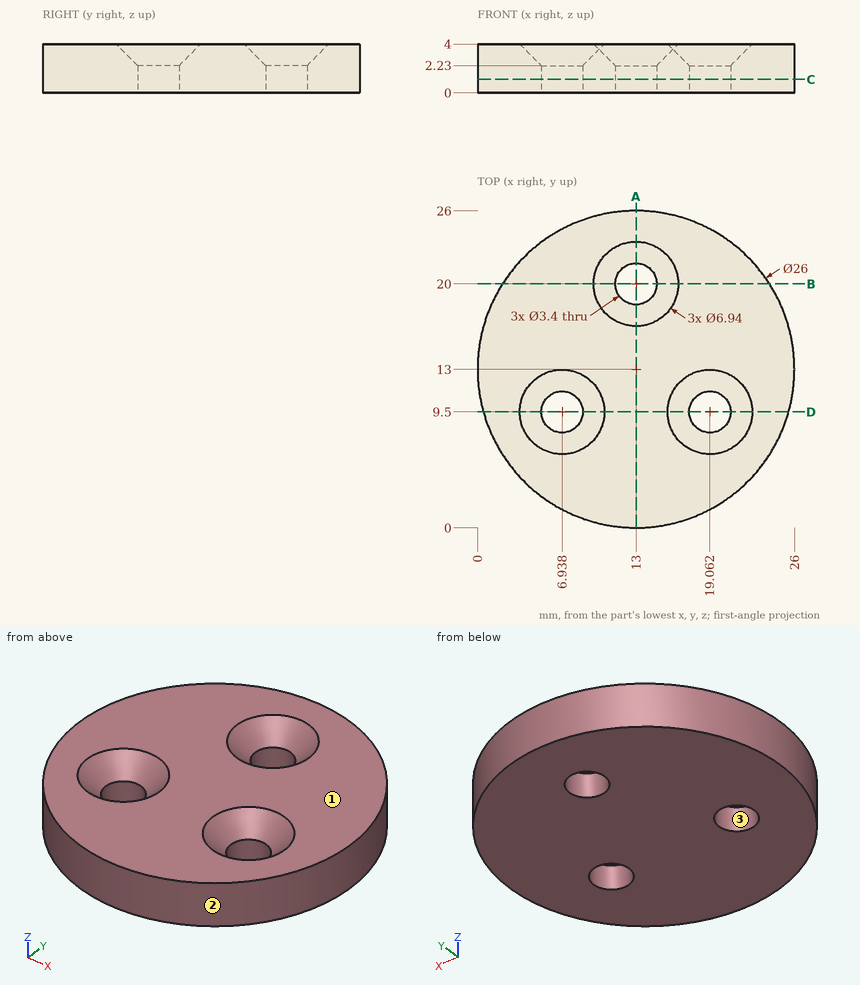
Verification items for this drawing (mm, ordinates from the low corner). Give positions to 0.01 mm unless a question says otherwise; leave off trailing zeros. Loops run counter-clockwise (first coordinate to the right, second up) from the corner with the lowest first, then second, coordinate; pieces in that order, holes last. Notation, with made-up numbers: M 28,43 L 78,43 A17 cw 78,54 Z; hole C 78,55 d2. An arc over 180 degrees is marked long. Answer as CSV lines item,"result".
Item 1: Release check for a two-part mould opening along Y. For the marked faces 1, 2 and 3 record: pulls with the +Y half, pulls with the -Y half, needs draft (parallel to the pull), parting line crosses it, or undercut.
Values:
face 1,"needs draft"
face 2,"parting line crosses it"
face 3,"undercut"
Item 2: Cross-section at D-D on y = 9.5. Record the cut outline in (x, z), and give its area (3 significant figures).
Values:
outline,"M 0.48,0 L 5.24,0 L 5.24,2.23 L 3.47,4 L 0.48,4 Z; M 8.64,0 L 17.36,0 L 17.36,2.23 L 15.59,4 L 10.41,4 L 8.64,2.23 Z; M 20.76,0 L 25.52,0 L 25.52,4 L 22.53,4 L 20.76,2.23 Z"
area,"66.7 mm²"
Item 3: Cross-section at C-C on z = 1.1. Record the cut outline in (x, y).
Values:
outline,"C 13,13 d26; hole C 6.94,9.5 d3.4; hole C 13,20 d3.4; hole C 19.06,9.5 d3.4"
Item 4: Cross-section at A-A on x = 13. Record the cut outline in (y, z).
Values:
outline,"M 0,0 L 18.3,0 L 18.3,2.23 L 16.53,4 L 0,4 Z; M 21.7,0 L 26,0 L 26,4 L 23.47,4 L 21.7,2.23 Z"
Item 5: Depth check by flat-ended pin: P1, Ø5.5, axis at x = 13, y = 20, coming from the -Z side. Enter the tip coordinate at first touch or a pass-through.
Values:
P1,"stops at z = 0"
Item 6: Material ranges on line 1 (X direction, y = 9.5, z = 1.15); line 2 (Y direction, x = 13, z = 1.25); line 3 (Y direction, x = 8.25, z = 2.45), recorded low to high.
Values:
line 1,"x = 0.48 to 5.24, 8.64 to 17.36, 20.76 to 25.52"
line 2,"y = 0 to 18.3, 21.7 to 26"
line 3,"y = 0.9 to 8.1, 10.9 to 25.1"
Item 7: Cross-section at B-B on y = 20. Record the cut outline in (x, z), and give its area (3 significant figures).
Values:
outline,"M 2.05,0 L 11.3,0 L 11.3,2.23 L 9.53,4 L 2.05,4 Z; M 14.7,0 L 23.95,0 L 23.95,4 L 16.47,4 L 14.7,2.23 Z"
area,"70.9 mm²"
